Check sheet for the modelled part. Datum: model origin and axes. Units: mm. A direction names the side the tool comes from. Round coordinates to 2 decimals unless told otherwise and drop trailing zeros. Loops run counter-clockwise (first coordinate to the right, second up) from the corner with the lowest first, then second, coordinate; pieces in that order, holes last. Notation, with made-up numbers: (80, -38) - (132, -38) arc R20 ccw to (132, -9) - close; hole circle Ø2 at (-15, -23). An arc over 180 degrees is marked (long way). Put each result on its own line as item: value. Start each with the question number.
```python
from build123d import *

# Parameters (mm, degrees)
BOSS_EXTRU_1_DEPTH = 5
ESQUISSE2_W        = 140
ESQUISSE2_H        = 5
BOSS_EXTRU_2_DEPTH = 5


with BuildPart() as part:
    # Esquisse1 → Boss.-Extru.1 (new body)
    with BuildSketch(Plane.XY):
        Polygon((85.505013729, -34.223744292), (85.505013729, -29.223744292), (-64.494986271, -29.223744292), (-64.494986271, -34.223744292), (-69.494986271, -34.223744292), (-69.494986271, -44.223744292), (-64.494986271, -44.223744292), (-64.494986271, -54.223744292), (-69.494986271, -54.223744292), (-69.494986271, -64.223744292), (-64.494986271, -64.223744292), (-64.494986271, -69.223744292), (85.505013729, -69.223744292), (85.505013729, -64.223744292), (90.505013729, -64.223744292), (90.505013729, -54.223744292), (85.505013729, -54.223744292), (85.505013729, -44.223744292), (90.505013729, -44.223744292), (90.505013729, -34.223744292), align=None)
    extrude(amount=BOSS_EXTRU_1_DEPTH)

    # Esquisse2 → Boss.-Extru.2 (add)
    with BuildSketch(Plane.XY.offset(5)):
        with Locations((10.505013729, -71.723744292)):
            Rectangle(ESQUISSE2_W, ESQUISSE2_H)
    extrude(amount=-BOSS_EXTRU_2_DEPTH)


solid = part.part
```
Q1. Material ranges on line 1 (X direction, y = -32, z = 0.3); line 2 (Y direction, x = -62, z = 4.5); line 3 (X direction, y = -70, z = 4.8), recorded low to high. Write a range as from..to.
Q2. Set-up check for faces 5 (the face through (-59.495, -72, 3)), 6 (the face through (-64.495, -49, 2)), 7 (the face through (88, -34.224, 2)), 8 (the face through (88, -44.224, 2)), 9 (the face through (85.505, -67, 2)): record each of +Z, -Z, +X, -X, +Y, -Y from which the full face is reachable in a straight line by a thin tool's end or side.
Q3. Depth check by flat-ended pin: pin 1 Ø2.5 at (y, z) = (-66, 1.5) entering from +X (3 decimals); pin 2 Ø2.5 at (x, z) = (87.5, 1.5) entering from +Y; pin 3 Ø2.5 at (x, z) = (88, 2) entering from -Y. Enter the tip coordinate at first touch or a pass-through.
Q4. Cross-section at A-A on z = 2.3. Enter the section's corners in (x, y).
Q5. Cross-section at B-B on y = -51. Enter the section's corners in (x, z), and give its area (3 significant figures).
Q6. Draft check along Y on faces 1 (the face through (85.505, -49, 2)), 2 (the face through (88, -54.224, 2)), 3 (the face through (-64.495, -67, 2)), 4 (the face through (-67, -34.224, 2)). Enter one of: +Y half, -Y half, draft (parallel to the pull), parting line (faces both ways), or undercut.
Q7. Cross-section at C-C on y = -71. Enter the section's corners in (x, z).
Answer list:
1. line 1: x = -64.49..85.51
1. line 2: y = -69.22..-29.22
1. line 3: x = -59.49..80.51
2. face 5: +Z, -Z, -X, -Y
2. face 6: +Z, -Z, -X
2. face 7: +Z, -Z, +X, +Y
2. face 8: +Z, -Z, +X
2. face 9: +Z, -Z, +X, -Y
3. pin 1: stops at x = 85.505
3. pin 2: stops at y = -34.22
3. pin 3: stops at y = -64.22
4. outline: (-69.49, -64.22) - (-64.49, -64.22) - (-64.49, -69.22) - (-59.49, -69.22) - (-59.49, -74.22) - (80.51, -74.22) - (80.51, -69.22) - (85.51, -69.22) - (85.51, -64.22) - (90.51, -64.22) - (90.51, -54.22) - (85.51, -54.22) - (85.51, -44.22) - (90.51, -44.22) - (90.51, -34.22) - (85.51, -34.22) - (85.51, -29.22) - (-64.49, -29.22) - (-64.49, -34.22) - (-69.49, -34.22) - (-69.49, -44.22) - (-64.49, -44.22) - (-64.49, -54.22) - (-69.49, -54.22) - close
5. outline: (-64.49, 0) - (85.51, 0) - (85.51, 5) - (-64.49, 5) - close
5. area: 750 mm2
6. face 1: undercut
6. face 2: undercut
6. face 3: draft
6. face 4: +Y half
7. outline: (-59.49, 0) - (80.51, 0) - (80.51, 5) - (-59.49, 5) - close
